Geometry: final body of the model. Coordinates: model frame, mm. A direction names the side the tool comes from. Give positions to 0.01 mm unless a question says otherwise; leave off trailing zeros. Write each loop counter-clockwise with the first axis right and the second up, starting at its lowest first coordinate (ties: lowest second). Pieces come first, ordered by that corner, then holes. Notation, with made-up numbers: M 46,-31.5 L 81,-31.5 A9 cw 81,-24.5 Z; hole C -37.75,4.5 d8. An arc over 180 degrees is marked long. Answer as a JSON object with one key per item and string values.
from build123d import *

# Parameters (mm, degrees)
SKETCH_1_R          = 4.35
EXTRUDE_1_DEPTH     = 3.45
SKETCH_2_R          = 0.715
EXTRUDE_2_DEPTH     = 2.3
SKETCH_3_R          = 2.85
CUT_EXTRUDE_1_DEPTH = 3.4
SKETCH_4_W          = 12.90394782
SKETCH_4_H          = 10.561384984
CUT_EXTRUDE_2_DEPTH = 10


with BuildPart() as part:
    # 草图1 → 凸台-拉伸1 (new body)
    with BuildSketch(Plane.XY):
        Circle(SKETCH_1_R)
    extrude(amount=EXTRUDE_1_DEPTH)

    # 草图2 → 凸台-拉伸2 (add)
    with BuildSketch(Plane.XY.offset(3.45)):
        with BuildLine():
            Line((-1.280487805, 5.861770294), (-16.933536585, 2.442404289))
            ThreePointArc((-16.933536585, 2.442404289), (-18.9, 0), (-16.933536585, -2.442404289))
            Line((-16.933536585, -2.442404289), (-1.280487805, -5.861770294))
            ThreePointArc((-1.280487805, -5.861770294), (0, -6), (1.280487805, -5.861770294))
            Line((1.280487805, -5.861770294), (16.933536585, -2.442404289))
            ThreePointArc((16.933536585, -2.442404289), (18.9, 0), (16.933536585, 2.442404289))
            Line((16.933536585, 2.442404289), (1.280487805, 5.861770294))
            ThreePointArc((1.280487805, 5.861770294), (0, 6), (-1.280487805, 5.861770294))
        make_face()
        with Locations((-16.4, 0)):
            Circle(SKETCH_2_R, mode=Mode.SUBTRACT)
        with Locations((-13.4, 0)):
            Circle(SKETCH_2_R, mode=Mode.SUBTRACT)
        with Locations((-10.4, 0)):
            Circle(SKETCH_2_R, mode=Mode.SUBTRACT)
        with Locations((-7.4, 0)):
            Circle(SKETCH_2_R, mode=Mode.SUBTRACT)
        with Locations((7.4, 0)):
            Circle(SKETCH_2_R, mode=Mode.SUBTRACT)
        with Locations((10.4, 0)):
            Circle(SKETCH_2_R, mode=Mode.SUBTRACT)
        with Locations((13.4, 0)):
            Circle(SKETCH_2_R, mode=Mode.SUBTRACT)
        with Locations((16.4, 0)):
            Circle(SKETCH_2_R, mode=Mode.SUBTRACT)
    extrude(amount=EXTRUDE_2_DEPTH)

    # 草图3 → 切除-拉伸1 (cut)
    with BuildSketch(Plane(origin=(0, 0, 0), x_dir=(-1, 0, 0), z_dir=(0, 0, -1))):
        Circle(SKETCH_3_R)
    extrude(amount=-CUT_EXTRUDE_1_DEPTH, mode=Mode.SUBTRACT)

    # 草图4 → 切除-拉伸2 (cut)
    with BuildSketch(Plane.XY.offset(5.75)):
        with Locations((18.45197391, -0.575714595)):
            Rectangle(SKETCH_4_W, SKETCH_4_H)
    extrude(amount=-CUT_EXTRUDE_2_DEPTH, mode=Mode.SUBTRACT)


solid = part.part
1) Cut plane B-B on y = 0. Give the number of separate pieces and of enclosed holes in the cut face, and give its area (3 significant figures).
Geometry check:
{"separate pieces": "7", "enclosed holes": "0", "area": "62.0 mm2"}
2) Contact query for flat-ended pins moving along their axis: P1, Ø1.1, axis at x = 7.4, y = 0, coming from the -Z side; P2, Ø1.5, axis at x = -14, y = 1, coming from the -Z side; P3, Ø1, axis at y = 0, z = 2, coming from the +X side; P4, Ø3, axis at x = 1.5, y = -1, coming from the -Z side. Output: stop coordinate, or through.
Geometry check:
{"P1": "passes through", "P2": "stops at z = 3.45", "P3": "stops at x = 4.35", "P4": "stops at z = 0"}
3) Pull-direction query (X, two-part tool) for faces 3 (the cylindrical face through (2.262, -1.734, 1.676)), 4 (the flat face through (12, 0, 5)), 5 (the flat face through (-9.217, -4.128, 4.584)); classes: pulls with the +X half, pulls with the -X half, needs draft (parallel to the pull), parting line crosses it, or undercut.
Geometry check:
{"face 3": "undercut", "face 4": "pulls with the +X half", "face 5": "pulls with the -X half"}
4) Cut plane D-D on x = 0. Return loops of the section in (y, z).
Geometry check:
{"outline": "M -6,3.45 L -4.35,3.45 L -4.35,0 L -2.85,0 L -2.85,3.4 L 2.85,3.4 L 2.85,0 L 4.35,0 L 4.35,3.45 L 6,3.45 L 6,5.75 L -6,5.75 Z"}
5) Cut plane A-A on x = -13.4. Return loops of the section in (y, z) (3 decimals), and give its area (3 significant figures).
Geometry check:
{"outline": "M -3.214,3.45 L -0.715,3.45 L -0.715,5.75 L -3.214,5.75 Z; M 0.715,3.45 L 3.214,3.45 L 3.214,5.75 L 0.715,5.75 Z", "area": "11.5 mm2"}
6) Line query: line 1 (Z direction, x = -9, y = 3); line 2 (X direction, y = 2, z = 0.6); line 3 (X direction, y = 1.25, z = 1.75). Output: solid intervals per line, ascending. Write a range as from..to.
Geometry check:
{"line 1": "z = 3.45..5.75", "line 2": "x = -3.86..-2.03, 2.03..3.86", "line 3": "x = -4.17..-2.56, 2.56..4.17"}
7) Cut plane C-C on z = 1.3. Return loops of the section in (x, y), and give its area (3 significant figures).
Geometry check:
{"outline": "C 0,0 d8.7; hole C 0,0 d5.7", "area": "33.9 mm2"}
8) Set-up query: faces 1 (the cylindrical face through (-12.718, 0.215, 4.584)), 2 (the flat face through (0, 0, 3.4)). Return all of +Z, -Z, +X, -X, +Y, -Y with unobstructed straight access to the full face (end or side cutting, diameter ignored); none if empty.
Geometry check:
{"face 1": "+Z, -Z", "face 2": "-Z"}
